Geometry: final body of the model. Coordinates: model frame, mm. A direction names the side the tool comes from. Give positions to 0.01 mm unless a question says otherwise; leave off trailing zeros. Write each loop counter-clockwise with the first axis right and the second up, starting at its lowest first coordinate (ties: lowest second). Pieces come first, ordered by that corner, then holes.
from build123d import *

# Parameters (mm, degrees)
SKETCH1_R           = 26.845
BOSS_EXTRUDE1_DEPTH = 6.23
SKETCH2_R           = 7.625
BOSS_EXTRUDE2_DEPTH = 700
SKETCH3_R           = 12.91
BOSS_EXTRUDE3_DEPTH = 12
SKETCH4_R           = 3.394618091
CUT_EXTRUDE1_DEPTH  = 12
CIRPATTERN1_COUNT   = 6
SKETCH6_R           = 6.26
BOSS_EXTRUDE4_DEPTH = 16.13


with BuildPart() as part:
    # Sketch1 → Boss-Extrude1 (new body)
    with BuildSketch(Plane(origin=(0, 0, 0), x_dir=(1, 0, 0), z_dir=(0, 1, 0))):
        with Locations(Location((0, 0, 0), (0, 0, 270))):
            Circle(SKETCH1_R)
    extrude(amount=BOSS_EXTRUDE1_DEPTH)

    # Sketch2 → Boss-Extrude2 (add)
    with BuildSketch(Plane(origin=(0, 6.23, 0), x_dir=(1, 0, 0), z_dir=(0, 1, 0))):
        with Locations(Location((0, 0, 0), (0, 0, 270))):
            Circle(SKETCH2_R)
    extrude(amount=BOSS_EXTRUDE2_DEPTH)

    # Sketch3 → Boss-Extrude3 (add)
    with BuildSketch(Plane.XZ):
        with Locations(Location((0, 0, 0), (0, 0, 90))):
            Circle(SKETCH3_R)
    extrude(amount=BOSS_EXTRUDE3_DEPTH)

    # Sketch4 → Cut-Extrude1 (cut)
    with BuildSketch(Plane(origin=(0, 0, 0), x_dir=(-1, 0, 0), z_dir=(0, -1, 0))):
        with Locations(Location((0, 18.718198498, 0), (0, 0, 90))):
            Circle(SKETCH4_R)
    cut_extrude1 = extrude(amount=-CUT_EXTRUDE1_DEPTH, mode=Mode.SUBTRACT)

    # CirPattern1: Cut-Extrude1 ×6 about axis
    cirpattern1_axis = Axis((0, 0, 0), (0, 1, 0))
    for i in range(1, CIRPATTERN1_COUNT):
        add(cut_extrude1.rotate(cirpattern1_axis, i * 360 / CIRPATTERN1_COUNT), mode=Mode.SUBTRACT)

    # Sketch6 → Boss-Extrude4 (add)
    with BuildSketch(Plane(origin=(0, -12, 0), x_dir=(-1, 0, 0), z_dir=(0, -1, 0))):
        with Locations(Location((0, 0, 0), (0, 0, 90))):
            Circle(SKETCH6_R)
    extrude(amount=BOSS_EXTRUDE4_DEPTH)


solid = part.part
Q1. Section B-B on y = 612.5. Output: boundary loops of the cut face in (x, z) (3 decimals).
Filled sheet:
outline: circle Ø15.25 at (0, 0)
Q2. Access query for faces 1 (the cylindrical face through (-6.1, -20, 1.4)), 2 (the flat face through (0, 706.23, 0)), 3 (the cylindrical face through (-7.444, 351.33, -1.653)). Directions: +Z, -Z, +X, -X, +Y, -Y. A direction counts if a zero-diameter tool reaches every point of the face in a straight line with its end or side. Return the directions, or none.
Filled sheet:
face 1: -Y
face 2: +Z, -Z, +X, -X, +Y
face 3: +Y
Q3. Pin query (flat end, axial travel): P1, Ø8, axis at x = 9.5, z = 5.5, coming from the -Y side; P2, Ø4, axis at x = 16.21, z = -9.36, coming from the +Y side; P3, Ø5, axis at x = -4, y = 588, coming from the -Z side; P4, Ø5, axis at y = 456, z = -1, coming from the -X side (3 decimals). Return the tip coordinate at first contact, or that it passes through.
Filled sheet:
P1: stops at y = -12
P2: passes through
P3: stops at z = -7.48
P4: stops at x = -7.625
Q4. Section A-A on z = 0. Output: boundary loops of the cut face in (x, y) (3 decimals).
Filled sheet:
outline: (-26.845, 0) - (-12.91, 0) - (-12.91, -12) - (-6.26, -12) - (-6.26, -28.13) - (6.26, -28.13) - (6.26, -12) - (12.91, -12) - (12.91, 0) - (26.845, 0) - (26.845, 6.23) - (7.625, 6.23) - (7.625, 706.23) - (-7.625, 706.23) - (-7.625, 6.23) - (-26.845, 6.23) - close
Q5. Ray query, line 1 along Y through (x, z) = (-13, 20); line 2 along Y through (x, z) = (2.5, 12.5); line 3 along X through (y, z) = (494, -0.5). Return the intervals inside material, ascending.
Filled sheet:
line 1: y = 0 to 6.23
line 2: y = -12 to 6.23
line 3: x = -7.61 to 7.61
